from build123d import *

# Parameters (mm, degrees)
F1_DEPTH = 63.5
F2_DEPTH = 7.9375
F3_DEPTH = 25.4
F0_W     = 25.4
F0_H     = 19.05
F4_DEPTH = 25.4
F6_R     = 5.08


# Not quite as in the source:
# - a feature names something its author has since deleted; it is built from what else it names


with BuildPart() as f1:
    # F0 (on Front) → F1 (new body, symmetric)
    with BuildSketch(Plane.XZ):
        Polygon((22.225, 9.525), (-41.275, 9.525), (-41.275, -9.525), (41.275, -9.525), (41.275, 9.525), align=None)
    extrude(amount=F1_DEPTH, both=True)

    # F0 (on Front) → F2 (join, symmetric)
    with BuildSketch(Plane.XZ):
        with BuildLine():
            add(Edge.make_bspline(
                [(-41.275, 9.525), (-41.6611139955, 40.1644010986), (17.1509007839, 61.4882749154), (56.5663251016, 61.9203224026)],
                knots=[0, 0, 0, 0, 110.9555033405, 110.9555033405, 110.9555033405, 110.9555033405], degree=3))
            Line((-41.275, 9.525), (22.225, 9.525))
            Line((22.225, 9.525), (22.225, 27.0002))
            ThreePointArc((22.225, 27.0002), (32.2487904829, 51.4886746276), (56.5663251016, 61.9203224026))
        make_face()
    extrude(amount=F2_DEPTH, both=True)

    # F0 (on Front) → F3 (join, symmetric)
    with BuildSketch(Plane.XZ):
        with BuildLine():
            Line((22.225, 27.0002), (22.225, 9.525))
            Line((22.225, 9.525), (41.275, 9.525))
            Line((41.275, 9.525), (41.275, 27.0002))
            ThreePointArc((41.275, 27.0002), (45.9246798487, 38.2255201513), (57.15, 42.8752))
            Line((57.15, 42.8752), (60.325, 42.8752))
            Line((60.325, 42.8752), (60.325, 61.9252))
            Line((60.325, 61.9252), (57.15, 61.9252))
            add(Edge.make_bspline(
                [(56.5663251016, 61.9203224026), (56.7613614994, 61.9224602709), (56.955922973, 61.9240866042), (57.15, 61.9252)],
                knots=[110.9555033405, 110.9555033405, 110.9555033405, 110.9555033405, 111.5045361635, 111.5045361635, 111.5045361635, 111.5045361635], degree=3))
            ThreePointArc((56.5663251016, 61.9203224026), (32.2487904829, 51.4886746276), (22.225, 27.0002))
        make_face()
    extrude(amount=F3_DEPTH, both=True)

    # F0 (on Front) → F4 (join, symmetric)
    with BuildSketch(Plane.XZ):
        with Locations((73.025, 52.4002)):
            Rectangle(F0_W, F0_H)
    extrude(amount=F4_DEPTH, both=True)

    # F0 (on Front) → F5 (revolve)
    with BuildSketch(Plane.XZ):
        Polygon((85.725, 66.675), (85.725, 61.9252), (85.725, 42.8752), (85.725, 38.1), (111.125, 38.1), (111.125, 66.675), align=None)
    revolve(axis=Axis((85.725, 0, 52.3875), (0, 0, 1)))

    # F6
    f6_edges = [f1.edges().sort_by_distance(p)[0] for p in [
        (-41.275, -63.5, 0),
        (41.275, -63.5, 0),
        (41.275, 63.5, 0),
        (-41.275, 63.5, 0),
    ]]
    fillet(f6_edges, radius=F6_R)


solid = f1.part
Model file for the job. Use its own axes, mm. A direction names the side the tool comes from. Give positions to 0.01 mm unless a question says otherwise; leave off trailing zeros. Write each loop counter-clockwise with the first axis right and the second up, starting at its lowest first coordinate (ties: lowest second). Pieces come first, ordered by that corner, then holes. Notation, with made-up numbers: (46.5, 48.5) -> (88.5, 48.5) arc R8 ccw to (88.5, 60.5) -> close; hole circle Ø3 at (51.5, 84.25). An arc over 180 degrees is marked (long way). Write item = value, one per line.
(1) Tool access for faces 1 (the face through (60, 2, 42.875)), 2 (the face through (-3, 7.938, 30)), 3 (the face through (46, 25.4, 42)), 4 (the face through (86, 0, 38.1)), 5 (the face through (-3, -7.938, 30)): list every direction of +Z, -Z, +X, -X, +Y, -Y with a clear straight run to the whole face (end or side of a thin tool).
Determined:
face_1 = -Z
face_2 = +Z, -X, +Y
face_3 = +Z, +X, -X, +Y
face_4 = -Z, +X, +Y, -Y
face_5 = +Z, -X, -Y
(2) Flat gauge pins, fed straight in: P1, Ø8.5, axis at x = 71.5, y = 2, coming from the -Z side; P2, Ø8, axis at y = 6.5, z = 48, coming from the -X side; P3, Ø5, axis at y = 18.5, z = 14.5, coming from the -X side (3 decimals); P4, Ø10, axis at x = 72.5, y = -34, coming from the -Z side. Where does each tip first touch, or does it go through?
Determined:
P1 = 38.1
P2 = -13.32
P3 = 22.225
P4 = through
(3) Probe line 1 along X through (y, z) = (-8.5, 1) (3 decimals); line 2 along Y through (x, z) = (-31, 24.5); line 3 along Z through (x, y) = (-15.5, -40.5) (3 decimals). List the from-to ranges inside material, lowest first.
Determined:
line_1 = -41.275 to 41.275
line_2 = -7.94 to 7.94
line_3 = -9.525 to 9.525
(4) Slice it at D-D, the plane x = 101.5. Give the cut face in (y, z) (3 decimals), then the cut area to 3 significant figures.
Determined:
outline = (-19.908, 38.1) -> (19.908, 38.1) -> (19.908, 66.675) -> (-19.908, 66.675) -> close
area = 1,140 mm2
(5) Slice it at B-B, the plane x = 65. Give the cut face in (y, z) (1 decimal).
Determined:
outline = (-25.4, 42.9) -> (-14.7, 42.9) -> (-14.7, 38.1) -> (14.7, 38.1) -> (14.7, 42.9) -> (25.4, 42.9) -> (25.4, 61.9) -> (14.7, 61.9) -> (14.7, 66.7) -> (-14.7, 66.7) -> (-14.7, 61.9) -> (-25.4, 61.9) -> close
(6) Slice it at A-A, the plane z = 5. Give the cut face in (x, y) (3 decimals).
Determined:
outline = (-41.275, -58.42) arc R5.08 ccw to (-36.195, -63.5) -> (36.195, -63.5) arc R5.08 ccw to (41.275, -58.42) -> (41.275, 58.42) arc R5.08 ccw to (36.195, 63.5) -> (-36.195, 63.5) arc R5.08 ccw to (-41.275, 58.42) -> close
(7) Slice it at C-C, the plane y = 30.5. Give the cut face in (x, z) (3 decimals).
Determined:
outline = (-41.275, -9.525) -> (41.275, -9.525) -> (41.275, 9.525) -> (-41.275, 9.525) -> close
(8) Mould opens along X. For faces 6 (the face through (45.8, -0.4, 38.1)), 7 (the face through (39.8, 62, 0.1)), 8 (the face through (1, 35, 9.525)) say: released by +X, released by -X, zero draft, split by the parting line, or undercut.
Determined:
face_6 = undercut
face_7 = released by +X
face_8 = zero draft
